Model file for the job. Use its own axes, mm. Give positions to 0.01 mm unless a question says otherwise; leave off trailing zeros. Write each loop counter-clockwise with the first axis right and the second up, starting at its lowest first coordinate (ties: lowest second). Pieces come first, ordered by that corner, then holes. Notation, with made-up numbers: (27, 12.25) - (37, 12.25) arc R29 cw to (37, 32.25) - close; hole circle Ø8 at (29.25, 37). An arc over 180 degrees is marked (long way). Use a Markdown table: item, result. Add a question column.
Autodesk Inventor part; units mm, degrees
ref_plane "YZ Plane" through (0, 0, 0) normal (1, 0, 0) x (0, 1, 0)
ref_plane "XZ Plane" through (0, 0, 0) normal (0, 1, 0) x (-1, 0, 0)
ref_plane "XY Plane" through (0, 0, 0) normal (0, 0, 1) x (1, 0, 0)
sketch "Sketch1" plane through (0, 0, 0) normal (1, 0, 0) x (0, 1, 0)
  line L0 (-26.5581, 0) -> (-13.2791, 23)
  line L1 (-13.2791, 23) -> (13.2791, 23)
  line L2 (13.2791, 23) -> (26.5581, 0)
  line L3 (26.5581, 0) -> (13.2791, -23)
  line L4 (13.2791, -23) -> (-13.2791, -23)
  line L5 (-13.2791, -23) -> (-26.5581, 0)
  point P0 (0, 0)
  point P1 (0, 0)
  dimension "d0" = 53.1162
extrude "Body" add sketch "Sketch1" along normal blind 24
sketch "Sketch2" plane through (0, 0, 0) normal (0, 0, 1) x (1, 0, 0)
  line L0 (0, 13.2791) -> (0, 26.5581)
  line L1 (0, 26.5581) -> (24, 26.5581)
  line L2 (24, 13.2791) -> (24, 26.5581)
  line L3 (-2.4, 0) -> (31.2, 0)
  line L4 (2.0543, 26.5581) -> (0, 23)
  line L5 (21.9457, 26.5581) -> (24, 23)
  dimension "d3" = 30
  dimension "d4" = 30
  dimension "d5" = 46
  dimension "d6" = 46
revolve "Chamfer1" cut sketch "Sketch2" angle 360 about axis through (-10, 0, 0) along (1, 0, 0)
sketch "Sketch3" plane through (24, 0, 0) normal (1, 0, 0) x (0, 0, -1)
  arc A0 (-11.5, -19.9186) -> (11.5, -19.9186) centre (0, 0) ccw
hole "Thread" at (24, 0, 0) direction (-1, 0, 0) diameter 26.211 end through all
chamfer "Chamfer2" distance 1.8944 angle 30 1 edges at (24, 0, 13.1055) measured on face at (24, 19.586, -0.5266)
chamfer "Chamfer3" distance 1.8944 angle 30 1 edges at (0, 0, 13.1055) measured on face at (0, 19.586, -0.5266)
equation "\"d0\" = 1.1547 * SW"
equation "\"d1\" = KOH"
equation "\"d3\" = ANG1"
equation "\"d4\" = ANG2"
equation "\"d5\" = SW0"
equation "\"d6\" = SW01"
equation "\"d8\" = -0.5 * GD1 + 0.5 * NND"
equation "\"d40\" = -0.5 * GD1 + 0.5 * NND"
equation "\"d10\" = -0.5 * GD1 + 0.5 * NND"
equation "\"d41\" = -0.5 * GD1 + 0.5 * NND"
equation "\"ANG1\" = 30deg"
equation "\"ANG2\" = ANG1"
equation "\"KOH\" = 24"
equation "\"SW\" = 46"
equation "\"SW0\" = SW"
equation "\"SW01\" = SW"
equation "\"TOA\" = 30deg"
equation "\"PTC\" = TPU"
equation "\"GAL\" = 0.541266 * TPU"
equation "\"GUL\" = 0.541266 * TPU"
equation "\"TPU\" = 3.5"
equation "\"E0\" = 1.155 * SW"
properties part number "BS 3692 - M30"
(1) Flat gauge pins, fed straight in: pin 1 (8 mm diameter, centred on x = 5, z = 17, fed in from +Y); pin 2 (3 mm diameter, centred on x = 10, y = -19.5, fed in from +Z); pin 3 (23.5 mm diameter, centred on y = 0, z = 0, fed in from +X); pin 4 (5 mm diameter, centred on x = 7, y = 16, fed in from -Z). Where does each tip first touch, or does it go through?
(2) Band-saw the part on A-A (x = 9.25). Write the cut outline in (y, z), then the cut area to 3 significant figures.
(3) Probe probe 1 along Y at (x, z) = (7.5, 0); probe 2 along Z at (x, y) = (18.5, 0); probe 3 along Y at (x, z) = (15.5, 20). List the from-to ranges inside material, lowest first. Write a range as [from, to].
(4) Two-plate mould, pull along Z, no slides. Class faces 1 (the conical face through (0.5, -11.98, -20.64)), 2 (the conical face through (23.5, 11.88, 20.7)), 3 (the conical face through (23.501, 23.865, 0.058)), 4 (the cylindrical face through (11.85, -3.94, -12.5)): +Z half, -Z half, draft (parallel to the pull), parting line (faces both ways), or undercut.
Model answer:
| question | item | result |
|---|---|---|
| 1 | pin 1 | stops at y = 19.05 |
| 1 | pin 2 | stops at z = 14.82 |
| 1 | pin 3 | passes through |
| 1 | pin 4 | stops at z = -22.62 |
| 2 | outline | (-26.56, 0) - (-13.28, -23) - (13.28, -23) - (26.56, 0) - (13.28, 23) - (-13.28, 23) - close; hole circle Ø26.21 at (0, 0) |
| 2 | area | 1,290 mm^2 |
| 3 | probe 1 | y = [-26.56, -13.11], [13.11, 26.56] |
| 3 | probe 2 | z = [-23, -13.11], [13.11, 23] |
| 3 | probe 3 | y = [-15.01, 15.01] |
| 4 | face 1 | -Z half |
| 4 | face 2 | +Z half |
| 4 | face 3 | parting line |
| 4 | face 4 | undercut |
